Autodesk Inventor part; units mm, degrees
ref_plane "Work Plane1" through (0, 0, -84) normal (0, 0, 1) x (1, 0, 0)
ref_plane "YZ Plane" through (0, 0, 0) normal (1, 0, 0) x (0, 1, 0)
ref_plane "XZ Plane" through (0, 0, 0) normal (0, 1, 0) x (-1, 0, 0)
sketch "Sketch1" plane through (0, 0, 0) normal (1, 0, 0) x (0, 1, 0)
  circle A0 centre (0, 0) radius 30
  line L0 (-30, 0) -> (-30, -130)
  line L1 (-30, -130) -> (30, -130)
  line L2 (30, -130) -> (30, 0)
  circle A1 centre (0, 0) radius 40
  line L3 (0, -50) -> (15, -50)
  line L4 (15, -50) -> (15, -85)
  line L5 (15, -85) -> (0, -85)
  line L6 (0, -85) -> (0, -50)
  point P0 (30, -26.4575)
  point P1 (-30, -26.4575)
  point P2 (0, -40)
  dimension "d16" = 80
  dimension "d0" = 60
  dimension "d1" = 130
  dimension "d18" = 30
  dimension "d19" = 45
  dimension "d20" = 10
  dimension "d21" = 35
extrude "Extrusion1" add sketch "Sketch1" along normal mid plane 55 contours L2 L1 L0 A1 | L3 L4 L5 L6
sketch "Sketch2" plane through (0, 0, 0) normal (0, 1, 0) x (-1, 0, 0)
  line L0 (27.5, -130) -> (-27.5, -130)
  circle A0 centre (0, -130) radius 46
  point P0 (0, 0)
  dimension "d4" = 92
extrude "Extrusion2" add sketch "Sketch2" along normal mid plane 60
ref_plane "Work Plane1" through (0, 0, -84) normal (0, 0, 1) x (1, 0, 0)
fillet "Fillet1" radius 10 2 edges at (0, 30, -26.4575) (0, -30, -26.4575)
sketch "Sketch3" plane through (0, 0, -84) normal (0, 0, 1) x (1, 0, 0)
  circle A0 centre (0, 0) radius 10
  dimension "d13" = 20
properties part number "thigh"
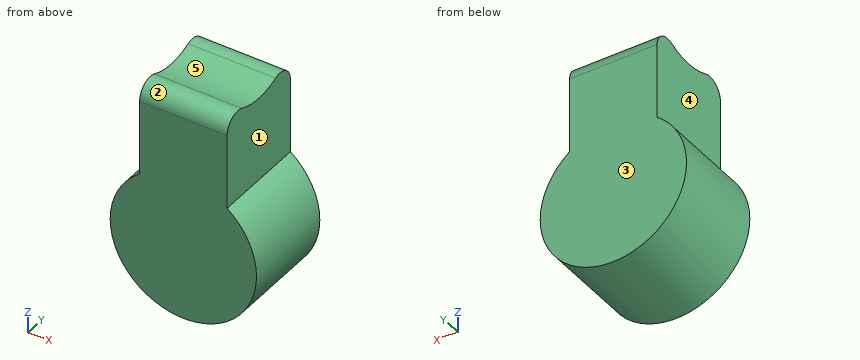
Work out the finished part from the listing and answer in its coordinate system (mm). Face numbers are marked on the shaded views. A direction names the side the tool comes from. Coordinates: 2 decimals unless noted, no trailing zeros. Loops run counter-clockwise (first coordinate to the right, second up) from the corner with the lowest first, then second, coordinate; pieces in that order, holes last. Notation, with made-up numbers: M 26.25,-10 L 76.25,-10 A19 ccw 76.25,10 Z; hole C -19.5,79 d9. An arc over 180 degrees is marked long. Answer in a Markdown table with one row per item. Add a question column.
1. Flat-ended cylindrical pins translate along their axes: P1, Ø5, axis at x = -22.5, y = -9, coming from the -Z side; P2, Ø8, axis at y = -6.5, z = -148.5, coming from the -X side; P3, Ø12, axis at x = 0, y = -6.5, coming from the -Z side. Find the tip coordinate at first contact, or state that the pin passes through.
2. Find section C-C, the plane y = 26. Write down the section's boundary in (x, z), then the cut area to 3 significant figures.
3. The mould has two halves that part along Y. Classify the marked faces 3, 4 and 5: pulls with the +Y half, pulls with the -Y half, needs draft (parallel to the pull), parting line crosses it, or undercut.
4. Find section A-A, the plane z = -76. Write down the section's boundary in (x, y), then the cut area to 3 significant figures.
5. A tool of negligible diameter and unlimited length cuts with its end or side. For the marked faces 1 and 2, from which of +Z, -Z, +X, -X, +Y, -Y can it reach the whole face along a straight path? Write none if from no direction.
6. Find section B-B, the plane x = 0. Write down the section's boundary in (y, z).
7. Consider L1, parallel to X at y = 3, z = -53.5; L2, parallel to X at y = 17.5, z = -130.5; L3, parallel to Z at x = 5, y = 27. Determine where each line is inside the solid, lowest interval first.
8. Find section D-D, the plane x = 23. Write down the section's boundary in (y, z).
Reported:
| question | item | result |
|---|---|---|
| 1 | P1 | stops at z = -171.42 |
| 1 | P2 | stops at x = -43.65 |
| 1 | P3 | stops at z = -176 |
| 2 | outline | M -27.5,-93.13 A46 ccw long 27.5,-93.13 L 27.5,-37.83 L -27.5,-37.83 Z |
| 2 | area | 9,350 mm^2 |
| 3 | face 3 | pulls with the +Y half |
| 3 | face 4 | needs draft |
| 3 | face 5 | undercut |
| 4 | outline | M -27.5,-30 L 27.5,-30 L 27.5,30 L -27.5,30 Z |
| 4 | area | 3,300 mm^2 |
| 5 | face 1 | +Z, +X, +Y, -Y |
| 5 | face 2 | +Z, +X, -X |
| 6 | outline | M -30,-176 L 30,-176 L 30,-45.83 A10 ccw 16,-36.66 A40 cw -16,-36.66 A10 ccw -30,-45.83 Z |
| 7 | L1 | x = -27.5 to 27.5 |
| 7 | L2 | x = -46 to 46 |
| 7 | L3 | z = -175.73 to -38.68 |
| 8 | outline | M -30,-169.84 L 30,-169.84 L 30,-45.83 A10 ccw 16,-36.66 A40 cw -16,-36.66 A10 ccw -30,-45.83 Z |
